Source: CAD feature listing. Evaluate the final solid. Frame: model axes, mm. A direction names the side the tool comes from. Round coordinates to 2 decimals unless told otherwise and drop trailing zeros. Loops run counter-clockwise (first coordinate to the right, second up) from the corner with the lowest first, then second, coordinate; pieces in that order, holes last. Notation, with made-up numbers: (-40, 26.25) -> (8, 26.25) arc R14 ccw to (8, 37.25) -> close; hole circle Ø8 at (-23, 87). An arc over 180 degrees is marked (long way). Put each result on its own line as item: value. Start each with the question number.
1. Contact query for flat-ended pins moving along their axis: pin 1 (1.5 mm diameter, centred on x = 283.5, z = 70, fed in from -Y); pin 2 (12 mm diameter, centred on x = 159.5, z = 80, fed in from +Y) (3 decimals); pin 3 (1.5 mm diameter, centred on x = 8, z = 220.5, fed in from +Y). Output: stop coordinate, or through.
2. Cut plane A-A (y = -125.5). Return the cut outline in (x, z), then the cut area to 3 significant figures.
3. Material intervals for L1, parallel to X at y = -168.5, z = 238; L2, parallel to Y at x = -70.5, z = -237; L3, parallel to Y at x = 231.5, z = 178, sorted ascending.
4. Set-up query: faces 1 (the cylindrical face through (-6.93, 81.137, -52.564)), 2 (the flat face through (499.93, 227.45, 142.65)), 3 (the flat face through (-495, 38, -137)). Return all of +Z, -Z, +X, -X, +Y, -Y with unobstructed straight access to the full face (end or side cutting, diameter ignored); none if empty.
5. Draft query along X for faces 4 (the cylindrical face through (-6.93, 71.92, -56.44)), 5 (the flat face through (505, 38, -124)), 6 (the flat face through (-499.93, 222.55, 151.135)). Return one class per face: pulls with the +X half, pulls with the -X half, needs draft (parallel to the pull), parting line crosses it, or undercut.
6. Cut plane D-D (y = 70.5). Return the cut outline in (x, z), then the cut area to 3 significant figures.
7. Cut plane B-B (z = 389.5). Return the cut outline in (x, y).
Autodesk Inventor part; units mm, degrees
ref_plane "YZ Plane" through (0, 0, 0) normal (1, 0, 0) x (0, 1, 0)
ref_plane "XZ Plane" through (0, 0, 0) normal (0, 1, 0) x (-1, 0, 0)
ref_plane "XY Plane" through (0, 0, 0) normal (0, 0, 1) x (1, 0, 0)
sketch "スケッチ1" plane through (0, 0, 0) normal (1, 0, 0) x (0, 1, 0)
  line L0 (10, 300) -> (0, 300)
  arc A0 (0, 300) -> (269.2388, -350) centre (919.2388, 300) ccw
  line L1 (0, -512.133) -> (0, 435.3555)
  arc A1 (10, 300) -> (276.3099, -342.9289) centre (919.2388, 300) ccw
  line L2 (-261.4236, 0) -> (1116.0159, 0)
  line L3 (276.3099, -342.9289) -> (269.2388, -350)
  point P0 (0, 0)
  dimension "d0" = 300
  dimension "d1" = 10
  dimension "d2" = 45
  dimension "d3" = 350
extrude "押し出し1" add sketch "スケッチ1" along normal mid plane 990 contours A1 L2 A0 L0 | A1 L3 A0 L2
sketch "スケッチ2" plane through (495, 0, 0) normal (1, 0, 0) x (0, 0, -1)
  line L0 (-450, 50) -> (-450, -200)
  line L1 (-450, -200) -> (500, -200)
  line L2 (500, -200) -> (500, 400)
  line L3 (500, 400) -> (156.2178, 400)
  line L4 (156.2178, 400) -> (-450, 50)
  line L5 (690, 0) -> (-640, 0)
  line L6 (-300, 10) -> (-300, 0)
  point P0 (0, 0)
  point P1 (350, 269.2388)
  dimension "d6" = 200
  dimension "d7" = 150
  dimension "d8" = 600
  dimension "d9" = 150
  dimension "d10" = 30
  dimension "d11" = 250
extrude "押し出し2" add sketch "スケッチ2" along normal blind 10
mirror "ミラー1" about plane through (0, 0, 0) normal (1, 0, 0) of "押し出し2"
properties part number "R-wing"
Solution:
1. pin 1: stops at y = 29.05
1. pin 2: stops at y = 38.535
1. pin 3: stops at y = 13.55
2. outline: (-505, -500) -> (-495, -500) -> (-495, 450) -> (-505, 450) -> close; (495, -500) -> (505, -500) -> (505, 450) -> (495, 450) -> close
2. area: 19,000 mm^2
3. L1: x = -505 to -495, 495 to 505
3. L2: y = 173.16 to 185.52
3. L3: y = 8.13 to 18.22
4. face 1: +Z, +Y
4. face 2: +Z, +X, -X, +Y
4. face 3: none
5. face 4: undercut
5. face 5: pulls with the +X half
5. face 6: needs draft
6. outline: (-505, -500) -> (-495, -500) -> (-495, -53.05) -> (495, -53.05) -> (495, -500) -> (505, -500) -> (505, 414.49) -> (495, 414.49) -> (495, -26.13) -> (-495, -26.13) -> (-495, 414.49) -> (-505, 414.49) -> close
6. area: 44,900 mm^2
7. outline: (-505, -200) -> (-495, -200) -> (-495, 84.93) -> (-505, 84.93) -> close; (495, -200) -> (505, -200) -> (505, 84.93) -> (495, 84.93) -> close
